CAD build for the part. Positions are in the model's coordinates, mm. Face numbers are marked on the shaded views. A direction names the side the tool comes from. Coordinates: 2 decimals unless noted, no trailing zeros. Loops run counter-clockwise (first coordinate to the right, second up) from the corner with the lowest first, then second, coordinate; pieces in that order, holes last. Notation, with made-up numbers: (-38, 71) -> (-15, 71) arc R31 cw to (-15, 97) -> close; hole circle Ø2 at (23, 47.25). An arc over 180 degrees is marked (long way). Answer as a JSON object with one key per item and string values. Group by question number.
from build123d import *

# Parameters (mm, degrees)
EXTRUDE_1_DEPTH     = 250
SKETCH_2_W          = 23
SKETCH_2_H          = 23
CUT_EXTRUDE_1_DEPTH = 26


with BuildPart() as part:
    # Эскиз1 → Вытянуть-Тонкостенный1 (new body)
    with BuildSketch(Plane(origin=(0, 0, 0), x_dir=(0, 0, -1), z_dir=(1, 0, 0))):
        Polygon((0, 25), (0, 0), (25, 0), (25, 2), (2, 2), (2, 25), align=None)
    extrude(amount=EXTRUDE_1_DEPTH)

    # Эскиз2 → Вырез-Вытянуть1 (cut, through all)
    with BuildSketch(Plane.XY):
        with Locations((238.5, 13.5)):
            Rectangle(SKETCH_2_W, SKETCH_2_H)
        with Locations((11.5, 13.5)):
            Rectangle(SKETCH_2_W, SKETCH_2_H)
    extrude(amount=-CUT_EXTRUDE_1_DEPTH, mode=Mode.SUBTRACT)


solid = part.part
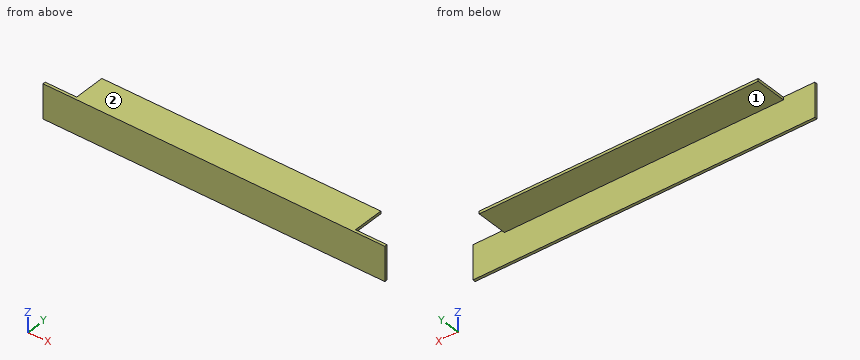
Item 1: 3-axis set-ups, long thin cutter, end or side, ignore diameter. For the marked faces 1 and 2: which of +Z, -Z, +X, -X, +Y, -Y reach the whole face in a straight line?
Item 2: Band-saw the part on C-C, the plane y = 5.75. List the corners of the cut face in (x, z), and give its area (3 significant figures).
Item 3: Band-saw the part on A-A, the plane x = 57. List the corners of the cut face in (y, z).
Item 4: Drill centre lines: L1, parallel to Z at x = 88.5, y = 18.5; L2, parallel to Y at x = 17, z = -19.5. Where is each one in solid material? Low to high.
Item 5: Flat gauge pins, fed straight in: P1, Ø4, axis at x = 176.5, z = -12.5, coming from the -Y side; P2, Ø5, axis at x = 66.5, y = 7, coming from the -Z side; P3, Ø1.5, axis at y = 22, z = -4, coming from the +X side; P4, Ø0.6, axis at y = 8, z = -1, coming from the -X side. Where does each tip first touch, or does it go through?
Item 6: Band-saw the part on B-B, the plane z = -17. List the corners of the cut face in (x, y), and give its area (3 significant figures).
Reply:
{
 "1": {"face 1": "-Z, +X, -X, +Y", "face 2": "+Z, +X, -X, +Y, -Y"},
 "2": {"outline": "(23, -2) -> (227, -2) -> (227, 0) -> (23, 0) -> close", "area": "408 mm²"},
 "3": {"outline": "(0, -25) -> (2, -25) -> (2, -2) -> (25, -2) -> (25, 0) -> (0, 0) -> close"},
 "4": {"L1": "-2 to 0", "L2": "0 to 2"},
 "5": {"P1": "y = 0", "P2": "z = -2", "P3": "through", "P4": "x = 23"},
 "6": {"outline": "(0, 0) -> (250, 0) -> (250, 2) -> (0, 2) -> close", "area": "500 mm²"}
}
